Job drawing, mm, ordinate dimensions from the low corner. One solid piece. A direction names the side the tool comes from. Round coordinates to 2 decimals unless told otherwise and drop trailing zeros. Write each loop counter-clockwise with the first axis right and the second up, starting at its lowest first coordinate (ties: lowest second). Pieces come first, ordered by that corner, then holes.
1) Saw through at B-B on x = 20. Write the cut outline in (y, z), and give its area (3 significant figures).
2) Drill centre lines: L1, parallel to Y at x = 20, z = 72; L2, parallel to Y at x = 16, z = 38; L3, parallel to Z at x = 4, y = 27.5. Where is each one in solid material? Low to high.
3) Which spindle directions (+Z, -Z, +X, -X, +Y, -Y) get a long thin tool onto all of the face, cutting with end or side? Do the marked faces 1 and 2. Say none if no direction does.
4) Flat gauge pins, fed straight in: pin 1 (1.5 mm diameter, centred on x = 20, y = 40, fed in from -Z); pin 2 (12 mm diameter, centred on x = 22.5, y = 38, fed in from -Z); pin 3 (20 mm diameter, centred on x = 15, z = 42.5, fed in from +Y). Where does each tip first touch, or does it go through?
5) Saw through at A-A on y = 40. Write the cut outline in (x, z), and give its area (4 significant figures).
6) Saw through at C-C on x = 11. Write the cut outline in (y, z), and give its area (3 significant figures).
7) Saw through at D-D on z = 54.5. Write the cut outline in (x, y), and give its area (3 significant figures).
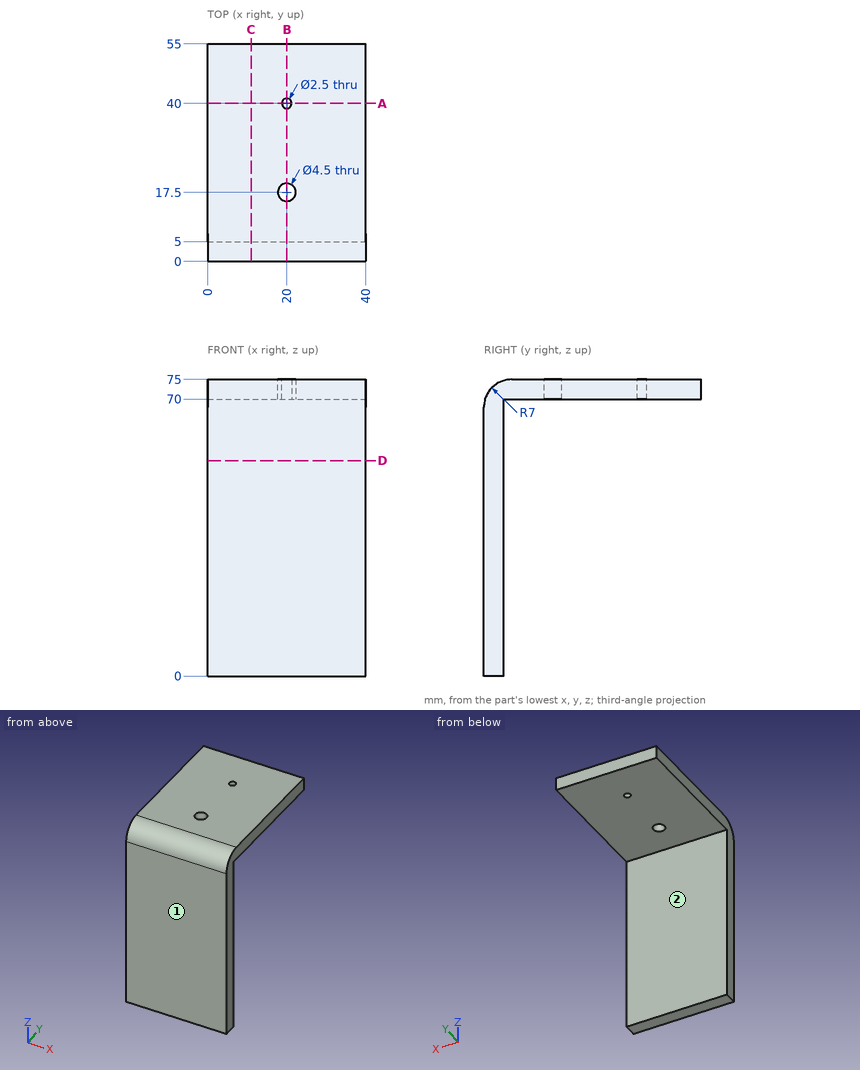
Completed:
1. outline: (0, 0) - (5, 0) - (5, 70) - (15.25, 70) - (15.25, 75) - (7, 75) arc R7 ccw to (0, 68) - close; (19.75, 70) - (38.75, 70) - (38.75, 75) - (19.75, 75) - close; (41.25, 70) - (55, 70) - (55, 75) - (41.25, 75) - close
1. area: 579 mm2
2. L1: y = 1.26 to 15.25, 19.75 to 38.75, 41.25 to 55
2. L2: y = 0 to 5
2. L3: z = 70 to 75
3. face 1: +Z, -Z, +X, -X, -Y
3. face 2: -Z, +X, -X, +Y
4. pin 1: passes through
4. pin 2: stops at z = 70
4. pin 3: stops at y = 5
5. outline: (0, 70) - (18.75, 70) - (18.75, 75) - (0, 75) - close; (21.25, 70) - (40, 70) - (40, 75) - (21.25, 75) - close
5. area: 187.5 mm2
6. outline: (0, 0) - (5, 0) - (5, 70) - (55, 70) - (55, 75) - (7, 75) arc R7 ccw to (0, 68) - close
6. area: 614 mm2
7. outline: (0, 0) - (40, 0) - (40, 5) - (0, 5) - close
7. area: 200 mm2
